from build123d import *

# Parameters (mm, degrees)
BOSS_EXTRUDE1_OUTLINE_W   = 296.4
BOSS_EXTRUDE1_OUTLINE_H   = 296.4
BOSS_EXTRUDE1_OUTLINE_W_2 = 20
BOSS_EXTRUDE1_OUTLINE_H_2 = 3.175
BOSS_EXTRUDE1_OUTLINE_W_3 = 3.175
BOSS_EXTRUDE1_OUTLINE_H_3 = 20
BOSS_EXTRUDE1_DEPTH       = 5.4
SKETCH3_W                 = 10
SKETCH3_H                 = 236.4
SKETCH3_W_2               = 236.4
SKETCH3_H_2               = 10
SKETCH3_W_3               = 80
SKETCH3_H_3               = 80
SKETCH3_H_4               = 175
SKETCH3_W_4               = 175
CUT_EXTRUDE5_DEPTH        = 10
SKETCH5_W                 = 296.48128
SKETCH5_H                 = 296.48128
SKETCH5_W_2               = 79.91872
SKETCH5_H_2               = 79.91872
SKETCH5_W_3               = 19.91872
SKETCH5_H_3               = 3.09372
SKETCH5_W_4               = 3.09372
SKETCH5_H_4               = 19.91872
BOSS_EXTRUDE2_DEPTH       = 5.4


# Read off the part's stored shape, not the designer's step: Boss-Extrude1
with BuildPart() as part:
    # Boss-Extrude1 outline → Boss-Extrude1 (new body)
    with BuildSketch(Plane(origin=(0, 0, 0), x_dir=(1, 0, 0), z_dir=(0, 1, 0))):
        with Locations((148.2, 148.2)):
            Rectangle(BOSS_EXTRUDE1_OUTLINE_W, BOSS_EXTRUDE1_OUTLINE_H)
        with BuildLine():
            Line((28.175, 5.025), (8.175, 5.025))
            ThreePointArc((8.175, 5.025), (5.92993597, 5.95493597), (5, 8.2))
            Line((5, 8.2), (5, 28.2))
            Line((5, 28.2), (8.175, 28.2))
            Line((8.175, 28.2), (8.175, 8.2))
            Line((8.175, 8.2), (28.175, 8.2))
            Line((28.175, 8.2), (28.175, 5.025))
        make_face(mode=Mode.SUBTRACT)
        with Locations((70.18, 6.6125)):
            Rectangle(BOSS_EXTRUDE1_OUTLINE_W_2, BOSS_EXTRUDE1_OUTLINE_H_2, mode=Mode.SUBTRACT)
        with Locations((6.5875, 70.205)):
            Rectangle(BOSS_EXTRUDE1_OUTLINE_W_3, BOSS_EXTRUDE1_OUTLINE_H_3, mode=Mode.SUBTRACT)
        with Locations((122.185, 6.6125)):
            Rectangle(BOSS_EXTRUDE1_OUTLINE_W_2, BOSS_EXTRUDE1_OUTLINE_H_2, mode=Mode.SUBTRACT)
        with Locations((6.5875, 122.21)):
            Rectangle(BOSS_EXTRUDE1_OUTLINE_W_3, BOSS_EXTRUDE1_OUTLINE_H_3, mode=Mode.SUBTRACT)
        with Locations((174.19, 6.6125)):
            Rectangle(BOSS_EXTRUDE1_OUTLINE_W_2, BOSS_EXTRUDE1_OUTLINE_H_2, mode=Mode.SUBTRACT)
        with Locations((226.195, 6.6125)):
            Rectangle(BOSS_EXTRUDE1_OUTLINE_W_2, BOSS_EXTRUDE1_OUTLINE_H_2, mode=Mode.SUBTRACT)
        with BuildLine():
            Line((291.375, 28.2), (291.375, 8.2))
            ThreePointArc((291.375, 8.2), (290.44506403, 5.95493597), (288.2, 5.025))
            Line((288.2, 5.025), (268.2, 5.025))
            Line((268.2, 5.025), (268.2, 8.2))
            Line((268.2, 8.2), (288.2, 8.2))
            Line((288.2, 8.2), (288.2, 28.2))
            Line((288.2, 28.2), (291.375, 28.2))
        make_face(mode=Mode.SUBTRACT)
        with Locations((289.7875, 70.205)):
            Rectangle(BOSS_EXTRUDE1_OUTLINE_W_3, BOSS_EXTRUDE1_OUTLINE_H_3, mode=Mode.SUBTRACT)
        with Locations((289.7875, 122.21)):
            Rectangle(BOSS_EXTRUDE1_OUTLINE_W_3, BOSS_EXTRUDE1_OUTLINE_H_3, mode=Mode.SUBTRACT)
        with Locations((6.5875, 174.215)):
            Rectangle(BOSS_EXTRUDE1_OUTLINE_W_3, BOSS_EXTRUDE1_OUTLINE_H_3, mode=Mode.SUBTRACT)
        with Locations((6.5875, 226.22)):
            Rectangle(BOSS_EXTRUDE1_OUTLINE_W_3, BOSS_EXTRUDE1_OUTLINE_H_3, mode=Mode.SUBTRACT)
        with BuildLine():
            Line((5, 268.225), (5, 288.225))
            ThreePointArc((5, 288.225), (5.92993597, 290.47006403), (8.175, 291.4))
            Line((8.175, 291.4), (28.175, 291.4))
            Line((28.175, 291.4), (28.175, 288.225))
            Line((28.175, 288.225), (8.175, 288.225))
            Line((8.175, 288.225), (8.175, 268.225))
            Line((8.175, 268.225), (5, 268.225))
        make_face(mode=Mode.SUBTRACT)
        with Locations((70.18, 289.8125)):
            Rectangle(BOSS_EXTRUDE1_OUTLINE_W_2, BOSS_EXTRUDE1_OUTLINE_H_2, mode=Mode.SUBTRACT)
        with Locations((122.185, 289.8125)):
            Rectangle(BOSS_EXTRUDE1_OUTLINE_W_2, BOSS_EXTRUDE1_OUTLINE_H_2, mode=Mode.SUBTRACT)
        with Locations((289.7875, 174.215)):
            Rectangle(BOSS_EXTRUDE1_OUTLINE_W_3, BOSS_EXTRUDE1_OUTLINE_H_3, mode=Mode.SUBTRACT)
        with Locations((174.19, 289.8125)):
            Rectangle(BOSS_EXTRUDE1_OUTLINE_W_2, BOSS_EXTRUDE1_OUTLINE_H_2, mode=Mode.SUBTRACT)
        with Locations((289.7875, 226.22)):
            Rectangle(BOSS_EXTRUDE1_OUTLINE_W_3, BOSS_EXTRUDE1_OUTLINE_H_3, mode=Mode.SUBTRACT)
        with Locations((226.195, 289.8125)):
            Rectangle(BOSS_EXTRUDE1_OUTLINE_W_2, BOSS_EXTRUDE1_OUTLINE_H_2, mode=Mode.SUBTRACT)
        with BuildLine():
            Line((268.2, 291.4), (288.2, 291.4))
            ThreePointArc((288.2, 291.4), (290.44506403, 290.47006403), (291.375, 288.225))
            Line((291.375, 288.225), (291.375, 268.225))
            Line((291.375, 268.225), (288.2, 268.225))
            Line((288.2, 268.225), (288.2, 288.225))
            Line((288.2, 288.225), (268.2, 288.225))
            Line((268.2, 288.225), (268.2, 291.4))
        make_face(mode=Mode.SUBTRACT)
    extrude(amount=BOSS_EXTRUDE1_DEPTH)

    # Sketch3 → Cut-Extrude5 (cut)
    with BuildSketch(Plane(origin=(0, 5.4, 0), x_dir=(1, 0, 0), z_dir=(0, 1, 0))):
        with BuildLine():
            ThreePointArc((24.475, 24.35), (19.475, 19.35), (14.475, 24.35))
            Line((14.475, 24.35), (24.475, 24.35))
        make_face()
        with Locations((19.475, 142.55)):
            Rectangle(SKETCH3_W, SKETCH3_H)
        with BuildLine():
            Line((24.475, 260.75), (14.475, 260.75))
            ThreePointArc((14.475, 260.75), (19.475, 265.75), (24.475, 260.75))
        make_face()
        with BuildLine():
            Line((35.65, 282.025), (35.65, 272.025))
            ThreePointArc((35.65, 272.025), (30.65, 277.025), (35.65, 282.025))
        make_face()
        with Locations((153.85, 277.025)):
            Rectangle(SKETCH3_W_2, SKETCH3_H_2)
        with BuildLine():
            ThreePointArc((272.05, 282.025), (277.05, 277.025), (272.05, 272.025))
            Line((272.05, 272.025), (272.05, 282.025))
        make_face()
        with Locations((75.675, 220.725)):
            Rectangle(SKETCH3_W_3, SKETCH3_H_3)
        with Locations((276.95, 123.2)):
            Rectangle(SKETCH3_W, SKETCH3_H_4)
        with BuildLine():
            Line((281.95, 210.7), (271.95, 210.7))
            ThreePointArc((271.95, 210.7), (276.95, 215.7), (281.95, 210.7))
        make_face()
        with BuildLine():
            ThreePointArc((281.95, 35.7), (276.95, 30.7), (271.95, 35.7))
            Line((271.95, 35.7), (281.95, 35.7))
        make_face()
        with BuildLine():
            ThreePointArc((260.7, 24.4), (265.7, 19.4), (260.7, 14.4))
            Line((260.7, 14.4), (260.7, 24.4))
        make_face()
        with Locations((173.2, 19.4)):
            Rectangle(SKETCH3_W_4, SKETCH3_H_2)
        with BuildLine():
            Line((85.7, 14.4), (85.7, 24.4))
            ThreePointArc((85.7, 24.4), (80.7, 19.4), (85.7, 14.4))
        make_face()
    extrude(amount=-CUT_EXTRUDE5_DEPTH, mode=Mode.SUBTRACT)

    # Sketch5 → Boss-Extrude2 (add)
    with BuildSketch(Plane(origin=(0, 5.4, 0), x_dir=(1, 0, 0), z_dir=(0, 1, 0))):
        with Locations((148.2, 148.2)):
            Rectangle(SKETCH5_W, SKETCH5_H)
        with BuildLine():
            Line((24.43436, 24.35), (24.43436, 260.75))
            ThreePointArc((24.43436, 260.75), (19.475, 265.70936), (14.51564, 260.75))
            Line((14.51564, 260.75), (14.51564, 24.35))
            ThreePointArc((14.51564, 24.35), (19.475, 19.39064), (24.43436, 24.35))
        make_face(mode=Mode.SUBTRACT)
        with Locations((75.675, 220.725)):
            Rectangle(SKETCH5_W_2, SKETCH5_H_2, mode=Mode.SUBTRACT)
        with BuildLine():
            Line((291.33436, 268.26564), (291.33436, 288.225))
            ThreePointArc((291.33436, 288.225), (290.416327211, 290.441327211), (288.2, 291.35936))
            Line((288.2, 291.35936), (268.24064, 291.35936))
            Line((268.24064, 291.35936), (268.24064, 288.26564))
            Line((268.24064, 288.26564), (288.24064, 288.26564))
            Line((288.24064, 288.26564), (288.24064, 268.26564))
            Line((288.24064, 268.26564), (291.33436, 268.26564))
        make_face(mode=Mode.SUBTRACT)
        with BuildLine():
            Line((268.24064, 5.06564), (288.2, 5.06564))
            ThreePointArc((288.2, 5.06564), (290.416327211, 5.983672789), (291.33436, 8.2))
            Line((291.33436, 8.2), (291.33436, 28.15936))
            Line((291.33436, 28.15936), (288.24064, 28.15936))
            Line((288.24064, 28.15936), (288.24064, 8.15936))
            Line((288.24064, 8.15936), (268.24064, 8.15936))
            Line((268.24064, 8.15936), (268.24064, 5.06564))
        make_face(mode=Mode.SUBTRACT)
        with BuildLine():
            Line((5.04064, 28.15936), (5.04064, 8.2))
            ThreePointArc((5.04064, 8.2), (5.958672789, 5.983672789), (8.175, 5.06564))
            Line((8.175, 5.06564), (28.13436, 5.06564))
            Line((28.13436, 5.06564), (28.13436, 8.15936))
            Line((28.13436, 8.15936), (8.13436, 8.15936))
            Line((8.13436, 8.15936), (8.13436, 28.15936))
            Line((8.13436, 28.15936), (5.04064, 28.15936))
        make_face(mode=Mode.SUBTRACT)
        with Locations((70.18, 289.8125)):
            Rectangle(SKETCH5_W_3, SKETCH5_H_3, mode=Mode.SUBTRACT)
        with Locations((122.185, 289.8125)):
            Rectangle(SKETCH5_W_3, SKETCH5_H_3, mode=Mode.SUBTRACT)
        with Locations((174.19, 289.8125)):
            Rectangle(SKETCH5_W_3, SKETCH5_H_3, mode=Mode.SUBTRACT)
        with Locations((226.195, 289.8125)):
            Rectangle(SKETCH5_W_3, SKETCH5_H_3, mode=Mode.SUBTRACT)
        with Locations((289.7875, 226.22)):
            Rectangle(SKETCH5_W_4, SKETCH5_H_4, mode=Mode.SUBTRACT)
        with Locations((289.7875, 174.215)):
            Rectangle(SKETCH5_W_4, SKETCH5_H_4, mode=Mode.SUBTRACT)
        with Locations((289.7875, 122.21)):
            Rectangle(SKETCH5_W_4, SKETCH5_H_4, mode=Mode.SUBTRACT)
        with Locations((289.7875, 70.205)):
            Rectangle(SKETCH5_W_4, SKETCH5_H_4, mode=Mode.SUBTRACT)
        with Locations((6.5875, 226.22)):
            Rectangle(SKETCH5_W_4, SKETCH5_H_4, mode=Mode.SUBTRACT)
        with Locations((6.5875, 174.215)):
            Rectangle(SKETCH5_W_4, SKETCH5_H_4, mode=Mode.SUBTRACT)
        with Locations((6.5875, 122.21)):
            Rectangle(SKETCH5_W_4, SKETCH5_H_4, mode=Mode.SUBTRACT)
        with Locations((6.5875, 70.205)):
            Rectangle(SKETCH5_W_4, SKETCH5_H_4, mode=Mode.SUBTRACT)
        with Locations((70.18, 6.6125)):
            Rectangle(SKETCH5_W_3, SKETCH5_H_3, mode=Mode.SUBTRACT)
        with Locations((122.185, 6.6125)):
            Rectangle(SKETCH5_W_3, SKETCH5_H_3, mode=Mode.SUBTRACT)
        with Locations((174.19, 6.6125)):
            Rectangle(SKETCH5_W_3, SKETCH5_H_3, mode=Mode.SUBTRACT)
        with Locations((226.195, 6.6125)):
            Rectangle(SKETCH5_W_3, SKETCH5_H_3, mode=Mode.SUBTRACT)
        with BuildLine():
            Line((271.99064, 210.7), (271.99064, 35.7))
            ThreePointArc((271.99064, 35.7), (276.95, 30.74064), (281.90936, 35.7))
            Line((281.90936, 35.7), (281.90936, 210.7))
            ThreePointArc((281.90936, 210.7), (276.95, 215.65936), (271.99064, 210.7))
        make_face(mode=Mode.SUBTRACT)
        with BuildLine():
            Line((5.04064, 288.225), (5.04064, 268.26564))
            Line((5.04064, 268.26564), (8.13436, 268.26564))
            Line((8.13436, 268.26564), (8.13436, 288.26564))
            Line((8.13436, 288.26564), (28.13436, 288.26564))
            Line((28.13436, 288.26564), (28.13436, 291.35936))
            Line((28.13436, 291.35936), (8.175, 291.35936))
            ThreePointArc((8.175, 291.35936), (5.958672789, 290.441327211), (5.04064, 288.225))
        make_face(mode=Mode.SUBTRACT)
        with BuildLine():
            Line((260.7, 24.35936), (85.7, 24.35936))
            ThreePointArc((85.7, 24.35936), (80.74064, 19.4), (85.7, 14.44064))
            Line((85.7, 14.44064), (260.7, 14.44064))
            ThreePointArc((260.7, 14.44064), (265.65936, 19.4), (260.7, 24.35936))
        make_face(mode=Mode.SUBTRACT)
        with BuildLine():
            Line((272.05, 281.98436), (35.65, 281.98436))
            ThreePointArc((35.65, 281.98436), (30.69064, 277.025), (35.65, 272.06564))
            Line((35.65, 272.06564), (272.05, 272.06564))
            ThreePointArc((272.05, 272.06564), (277.00936, 277.025), (272.05, 281.98436))
        make_face(mode=Mode.SUBTRACT)
    extrude(amount=-BOSS_EXTRUDE2_DEPTH)


solid = part.part
Read the model definition and answer for the solid it produces. Units are mm, in the model's axes. Coordinates: 2 decimals unless noted, no trailing zeros. Order: outer loops, then holes, each group sorted by start corner. A loop starts at its lowest first (then second) coordinate and runs counter-clockwise, first axis right, second up. Notation, with made-up numbers: M 46.5,-29.75 L 96.5,-29.75 A27 ccw 96.5,6.25 Z; hole C -14.75,-5 d7. An arc over 180 degrees is marked long. Put each result on its own line as item: value. Start each with the question number.
Item 1: Section C-C, the plane z = -226 is taken. Determine the outline of the cut face in (x, y).
Item 2: Section D-D, the plane y = 2.8 is taken. Count the separate pieces of the cut face and the enclosed holes in it, plus the area to 3 significant figures.
Item 3: Consider probe 1 along X at (y, z) = (0.6, -247.5); probe 2 along Z at (x, y) = (184.5, 4.4); probe 3 along X at (y, z) = (3.6, -73). Determine where each line is inside the solid, lowest interval first. Write a range as [from, to].
Item 4: Section A-A, the plane x = 53 is taken. Determine the outline of the cut face in (y, z).
Item 5: Given pin 1 Ø3 at (x, z) = (264.5, -77) entering from -Y, flat-ended and moving along its own axis, determine where the tip first touches the part or whether it passes through.
Item 6: Section B-B, the plane x = 104 is taken. Determine the outline of the cut face in (y, z).
Computed:
1. outline: M -0.04,0 L 5.04,0 L 5.04,5.4 L -0.04,5.4 Z; M 8.13,0 L 14.52,0 L 14.52,5.4 L 8.13,5.4 Z; M 24.43,0 L 35.72,0 L 35.72,5.4 L 24.43,5.4 Z; M 115.63,0 L 288.24,0 L 288.24,5.4 L 115.63,5.4 Z; M 291.33,0 L 296.44,0 L 296.44,5.4 L 291.33,5.4 Z
2. separate pieces: 1
2. enclosed holes: 25
2. area: 71,500 mm2
3. probe 1: x = [-0.04, 14.52], [24.43, 35.72], [115.63, 296.44]
3. probe 2: z = [-296.44, -281.98], [-272.07, -24.36], [-14.44, 0.04]
3. probe 3: x = [-0.04, 5.04], [8.13, 14.52], [24.43, 271.99], [281.91, 288.24], [291.33, 296.44]
4. outline: M 0,-296.44 L 5.4,-296.44 L 5.4,-281.98 L 0,-281.98 Z; M 0,-272.07 L 5.4,-272.07 L 5.4,-260.68 L 0,-260.68 Z; M 0,-180.77 L 5.4,-180.77 L 5.4,0.04 L 0,0.04 Z
5. pin 1: stops at y = 0
6. outline: M 0,-296.44 L 5.4,-296.44 L 5.4,-281.98 L 0,-281.98 Z; M 0,-272.07 L 5.4,-272.07 L 5.4,-260.68 L 0,-260.68 Z; M 0,-180.77 L 5.4,-180.77 L 5.4,-24.36 L 0,-24.36 Z; M 0,-14.44 L 5.4,-14.44 L 5.4,0.04 L 0,0.04 Z
